from build123d import *

# Parameters (mm, degrees)
SKETCH1_W           = 170
SKETCH1_H           = 50
SKETCH1_R           = 2.5
BOSS_EXTRUDE1_DEPTH = 5


with BuildPart() as part:
    # Sketch1 → Boss-Extrude1 (new body)
    with BuildSketch(Plane(origin=(0, 0, 0), x_dir=(1, 0, 0), z_dir=(0, 1, 0))):
        Rectangle(SKETCH1_W, SKETCH1_H)
        with Locations((74, 11)):
            Circle(SKETCH1_R, mode=Mode.SUBTRACT)
        with Locations((52, 11)):
            Circle(SKETCH1_R, mode=Mode.SUBTRACT)
        with Locations((52, -11)):
            Circle(SKETCH1_R, mode=Mode.SUBTRACT)
        with Locations((74, -11)):
            Circle(SKETCH1_R, mode=Mode.SUBTRACT)
        with Locations((26, 11)):
            Circle(SKETCH1_R, mode=Mode.SUBTRACT)
        with Locations((4, 11)):
            Circle(SKETCH1_R, mode=Mode.SUBTRACT)
        with Locations((4, -11)):
            Circle(SKETCH1_R, mode=Mode.SUBTRACT)
        with Locations((26, -11)):
            Circle(SKETCH1_R, mode=Mode.SUBTRACT)
        with Locations((-51, 11)):
            Circle(SKETCH1_R, mode=Mode.SUBTRACT)
        with Locations((-73, 11)):
            Circle(SKETCH1_R, mode=Mode.SUBTRACT)
        with Locations((-51, -11)):
            Circle(SKETCH1_R, mode=Mode.SUBTRACT)
        with Locations((-73, -11)):
            Circle(SKETCH1_R, mode=Mode.SUBTRACT)
    extrude(amount=BOSS_EXTRUDE1_DEPTH)


solid = part.part
Read the model definition and answer for the solid it produces. Units are mm, in the model's axes. Give positions to 0.01 mm unless a question says otherwise; leave off trailing zeros. Write each loop counter-clockwise with the first axis right and the second up, starting at its lowest first coordinate (ties: lowest second). Pieces come first, ordered by that corner, then holes. Notation, with made-up numbers: (-40, 59) - (-29, 59) arc R29 ccw to (-29, 95) - close; hole circle Ø8 at (38.5, -7). An arc over 180 degrees is marked (long way). Use CSV: the item, a comma, the result in double quotes. Start each with the question number.
Item 1: The mould has two halves that part along Z. Classify faces 1 (the cylindrical face through (3.46, 2.46, 13.44)), 2 (the flat face through (-1, 5, 0)), 3 (the flat face through (-1, 2, -25)): pulls with the +Z half, pulls with the -Z half, needs draft (parallel to the pull), parting line crosses it, or undercut.
Item 2: A flat-ended cylindrical pin translates along its axis: P1, Ø4, axis at x = 26, z = -11, coming from the -Y side (3 decimals). Find the tip coordinate at first contact, or state that the pin passes through.
Item 3: The part is cut by section A-A, the plane y = 1.1. Count the separate pieces of the cut face and the enclosed holes in it, and give its area (3 significant figures).
Item 4: Consider line 1 (Z direction, x = 74, y = 3.55); line 2 (Z direction, x = 5.5, y = 3.7). Determine where each line is inside the solid, lowest interval first.
Item 5: The part is cut by section C-C, the plane x = 4. Give the vertices of the cut face in (y, z).
Item 6: The part is cut by section B-B, the plane z = 11. Give the vertices of the cut face in (x, y).
Taken from the geometry:
1,face 1,"undercut"
1,face 2,"needs draft"
1,face 3,"pulls with the -Z half"
2,P1,"through"
3,separate pieces,"1"
3,enclosed holes,"12"
3,area,"8,260 mm2"
4,line 1,"-25 to -13.5, -8.5 to 8.5, 13.5 to 25"
4,line 2,"-25 to -13, -9 to 9, 13 to 25"
5,outline,"(0, -25) - (5, -25) - (5, -13.5) - (0, -13.5) - close; (0, -8.5) - (5, -8.5) - (5, 8.5) - (0, 8.5) - close; (0, 13.5) - (5, 13.5) - (5, 25) - (0, 25) - close"
6,outline,"(-85, 0) - (-75.5, 0) - (-75.5, 5) - (-85, 5) - close; (-70.5, 0) - (-53.5, 0) - (-53.5, 5) - (-70.5, 5) - close; (-48.5, 0) - (1.5, 0) - (1.5, 5) - (-48.5, 5) - close; (6.5, 0) - (23.5, 0) - (23.5, 5) - (6.5, 5) - close; (28.5, 0) - (49.5, 0) - (49.5, 5) - (28.5, 5) - close; (54.5, 0) - (71.5, 0) - (71.5, 5) - (54.5, 5) - close; (76.5, 0) - (85, 0) - (85, 5) - (76.5, 5) - close"
